Design review of the part built by this model. Coordinates are the model's own, in mm. A direction names the side the tool comes from. Coordinates: 2 decimals unless noted, no trailing zeros. Loops run counter-clockwise (first coordinate to the right, second up) from the corner with the lowest first, then second, coordinate; pieces in that order, holes last. Notation, with made-up numbers: M -19.5,-11 L 16.5,-11 A20 cw 16.5,4 Z; hole C -10,20.5 d1. An arc over 180 degrees is marked long. Put each result on its own line as item: value. Start each with the question number.
(1) For faces 1 (the flat face through (480.04, 662.21, 23.37)), 2 (the flat face through (485.032, 662.664, 13.664)), 3 (the flat face through (505.304, 661.264, 47.407)), list the 3-axis set-ups (+Z, -Z, +X, -X, +Y, -Y) from which the entire face can be reached by the end or side of a thin tool; tool diameter is ignored.
(2) For probe 1 along Z at (x, y) = (485.5, 661.5); probe 2 along Z at (x, y) = (490.5, 664.25); probe 3 along Z at (x, y) = (500, 662.75), list the stretches that pass through material, from the lowest coordinate up. Write a range as [from, to].
(3) Take a section at A-A, the plane z = 40.5. Give the boundary of the cut face in (x, y).
(4) Take a section at C-C, the plane x = 503.5. Give the boundary of the cut face in (y, z), then the cut area to 3 significant figures.
(5) Take a section at B-B, the plane z = 50. Give the boundary of the cut face in (x, y).
(6) Clearance check with flat-ended pins moving along their axes: pin 1 (1.5 mm diameter, centred on x = 480.5, y = 660.5, fed in from -Z); pin 2 (2 mm diameter, centred on y = 667.5, z = 54.5, fed in from +X); pin 3 (6 mm diameter, centred on x = 539, y = 663.5, fed in from +Z). State where each tip first meets the part, or that it passes through.
(7) The part is to be moulded in two halves that separate along X. For faces 4 (the cylindrical face through (547.15, 668.28, 45.1)), 5 (the flat face through (483.68, 662.54, 89.1)), 6 (the flat face through (484.08, 662.578, 70.684)), say which applies: +X half, -X half, draft (parallel to the pull), parting line (faces both ways), or undercut.
(8) Take a section at D-D, the plane z = 10. Give the boundary of the cut face in (x, y), then the cut area to 3 significant figures.
```python
from build123d import *

# Parameters (mm, degrees)
SKETCH1_R           = 12.573
SKETCH1_R_2         = 9.398
BOSS_EXTRUDE1_DEPTH = 3.175
FILLET1_R           = 12.7


with BuildPart() as part:
    # Sketch1 → Boss-Extrude1 (new body, symmetric)
    with BuildSketch(Plane(origin=(-54.155377654, 613.87875058, 32.992743825), x_dir=(0, 0, 1), z_dir=(-0.090029847, 0.995939068, 0))):
        with BuildLine():
            Line((1.896014785, 593.288148249), (-29.623565633, 535.82564653))
            Line((-29.623565633, 535.82564653), (-24.056128994, 532.771772062))
            Line((-24.056128994, 532.771772062), (-14.466963164, 550.253523109))
            ThreePointArc((-14.466963164, 550.253523109), (-7.052635612, 552.415186576), (-4.890972145, 545.000859024))
            Line((-4.890972145, 545.000859024), (-14.480137975, 527.519107976))
            Line((-14.480137975, 527.519107976), (-8.912701335, 524.465233508))
            Line((-8.912701335, 524.465233508), (14.368665453, 566.908868904))
            Line((14.368665453, 566.908868904), (3.548423472, 584.90983519))
            ThreePointArc((3.548423472, 584.90983519), (1.989104795, 588.954403604), (1.896014785, 593.288148249))
        make_face()
        with BuildLine():
            ThreePointArc((22.606879083, 581.927735227), (12.380822619, 578.965387193), (3.548423472, 584.90983519))
            Line((3.548423472, 584.90983519), (14.368665453, 566.908868904))
            Line((14.368665453, 566.908868904), (22.606879083, 581.927735227))
        make_face()
        with BuildLine():
            Line((58.865434837, 541.692100135), (25.100547859, 597.864650913))
            ThreePointArc((25.100547859, 597.864650913), (26.43992538, 594.748262171), (26.897485666, 591.387243051))
            ThreePointArc((26.897485666, 591.387243051), (25.774700979, 586.193699148), (22.606879083, 581.927735227))
            Line((22.606879083, 581.927735227), (14.368665453, 566.908868904))
            Line((14.368665453, 566.908868904), (37.31331045, 528.737284412))
            Line((37.31331045, 528.737284412), (42.755766103, 532.008702524))
            Line((42.755766103, 532.008702524), (32.483513232, 549.098013274))
            ThreePointArc((32.483513232, 549.098013274), (34.611130022, 557.637609564), (43.150726312, 555.509992774))
            Line((43.150726312, 555.509992774), (53.422979184, 538.420682023))
            Line((53.422979184, 538.420682023), (58.865434837, 541.692100135))
        make_face()
        with Locations((14.324485666, 591.387243051)):
            Circle(SKETCH1_R)
        with Locations((14.324485666, 591.387243051)):
            Circle(SKETCH1_R_2, mode=Mode.SUBTRACT)
    extrude(amount=BOSS_EXTRUDE1_DEPTH, both=True)

    # Fillet1
    fillet1_edges = [part.edges().sort_by_distance(p)[0] for p in [
        (510.451312753, 664.917469113, 47.361409278),
    ]]
    fillet(fillet1_edges, radius=FILLET1_R)


solid = part.part
```
Computed values:
1. face 1: +Y
1. face 2: -X, -Y
1. face 3: +Z, -Z, +X, -Y
2. probe 1: z = [6.62, 13.86], [26.32, 33.56], [62.48, 69.89], [84.41, 91.82]
2. probe 2: z = [9.49, 16.73], [28.74, 36.43], [59.34, 66.75], [81.27, 88.68]
2. probe 3: z = [14.6, 66.04], [75.58, 83.07]
3. outline: M 495.08,666.72 L 495.66,660.39 L 528.67,663.38 L 528.1,669.7 Z; M 540.99,670.87 L 541.56,664.54 L 545.64,664.91 L 545.07,671.23 Z
4. outline: M 661.1,16.43 L 667.48,16.75 L 667.48,80.72 L 661.1,81.07 Z
4. area: 410 mm^2
5. outline: M 497.25,666.91 L 497.82,660.59 L 526.15,663.15 L 525.57,669.47 Z; M 543.51,671.09 L 544.09,664.77 L 547.35,665.07 L 546.78,671.39 Z
6. pin 1: stops at z = 3.43
6. pin 2: stops at x = 545.8
6. pin 3: stops at z = 61.42
7. face 4: +X half
7. face 5: -X half
7. face 6: undercut
8. outline: M 478.1,665.18 L 478.67,658.86 L 491.82,660.05 L 491.25,666.37 Z
8. area: 83.8 mm^2
